Here's how the part is built. I have some questions about the finished solid (model axes, mm). A direction names the side the tool comes from. Give positions to 0.01 mm unless a question says otherwise; leave off trailing zeros. Write each loop counter-clockwise with the first axis right and the second up, starting at its lowest first coordinate (ties: lowest second). Pieces come first, ordered by that corner, then holes. Notation, with made-up numbers: (-5.5, 42) - (50.5, 42) arc R19 cw to (50.5, 60) - close; hole circle Ø9 at (36, 22). An arc over 180 degrees is marked (long way). Use a Markdown table: item, result.
```python
from build123d import *

# Parameters (mm, degrees)
F1_DEPTH  = 270
F2_W      = 88
F2_H      = 212
F3_DEPTH  = 178
F4_W      = 68
F4_H      = 172
F5_DEPTH  = 5
F7_DEPTH  = 128
F8_W      = 42
F8_H      = 66
F9_DEPTH  = 163
F11_DEPTH = 146


with BuildPart() as f1:
    # F0 (on Front) → F1 (new body)
    with BuildSketch(Plane.XZ):
        with BuildLine():
            Line((-20, 505), (-665, 505))
            ThreePointArc((-665, 505), (-679.142136, 499.142136), (-685, 485))
            Line((-685, 485), (-685, 20))
            ThreePointArc((-685, 20), (-679.142136, 5.857864), (-665, 0))
            Line((-665, 0), (-20, 0))
            ThreePointArc((-20, 0), (-5.857864, 5.857864), (0, 20))
            Line((0, 20), (0, 485))
            ThreePointArc((0, 485), (-5.857864, 499.142136), (-20, 505))
        make_face()
    extrude(amount=-F1_DEPTH)

    # F2 (on face) → F3 (cut)
    with BuildSketch(Plane.XZ):
        with Locations((-541.250854, 142.595568)):
            Rectangle(F2_W, F2_H)
    extrude(amount=-F3_DEPTH, mode=Mode.SUBTRACT)

    # F4 (on face) → F5 (cut)
    with BuildSketch(Plane.XZ.offset(-178)):
        with Locations((-541.250854, 142.595568)):
            Rectangle(F4_W, F4_H)
    extrude(amount=-F5_DEPTH, mode=Mode.SUBTRACT)

    # F6 (on face) → F7 (cut)
    with BuildSketch(Plane.XZ):
        with BuildLine():
            Line((-456.298642, 342.595568), (-456.298642, 36.595568))
            Line((-456.298642, 36.595568), (-279.298642, 36.595568))
            Line((-279.298642, 36.595568), (-271.298642, 36.595568))
            ThreePointArc((-271.298642, 36.595568), (-269.884428, 37.181354), (-269.298642, 38.595568))
            Line((-269.298642, 38.595568), (-269.298642, 61.595568))
            ThreePointArc((-269.298642, 61.595568), (-269.884428, 63.009782), (-271.298642, 63.595568))
            Line((-271.298642, 63.595568), (-277.298642, 63.595568))
            ThreePointArc((-277.298642, 63.595568), (-278.712855, 64.181354), (-279.298642, 65.595568))
            Line((-279.298642, 65.595568), (-279.298642, 313.595568))
            ThreePointArc((-279.298642, 313.595568), (-278.712855, 315.009782), (-277.298642, 315.595568))
            Line((-277.298642, 315.595568), (-271.298642, 315.595568))
            ThreePointArc((-271.298642, 315.595568), (-269.884428, 316.181354), (-269.298642, 317.595568))
            Line((-269.298642, 317.595568), (-269.298642, 340.595568))
            ThreePointArc((-269.298642, 340.595568), (-269.884428, 342.009782), (-271.298642, 342.595568))
            Line((-271.298642, 342.595568), (-317.298642, 342.595568))
            Line((-317.298642, 342.595568), (-317.298642, 402.595568))
            ThreePointArc((-317.298642, 402.595568), (-320.227574, 409.666636), (-327.298642, 412.595568))
            Line((-327.298642, 412.595568), (-396.298642, 412.595568))
            ThreePointArc((-396.298642, 412.595568), (-403.36971, 409.666636), (-406.298642, 402.595568))
            Line((-406.298642, 402.595568), (-406.298642, 342.595568))
            Line((-406.298642, 342.595568), (-456.298642, 342.595568))
        make_face()
    extrude(amount=-F7_DEPTH, mode=Mode.SUBTRACT)

    # F8 (on face) → F9 (cut)
    with BuildSketch(Plane.XZ):
        with Locations((-171, 68.898773)):
            Rectangle(F8_W, F8_H)
    extrude(amount=-F9_DEPTH, mode=Mode.SUBTRACT)

    # F10 (on face) → F11 (cut)
    with BuildSketch(Plane.XZ):
        Polygon((-192, 275.058829), (-192, 176.058829), (-138, 176.058829), (-138, 206.058829), (-158, 206.058829), (-158, 275.058829), align=None)
    extrude(amount=-F11_DEPTH, mode=Mode.SUBTRACT)


solid = f1.part
```
Item 1: For faces 4 (the cylindrical face through (-678.986, 133.11, 499.297)), 5 (the flat face through (-406.299, 63, 373)), which set-ups out of +Z, -Z, +X, -X, +Y, -Y let a thin tool reach every point of the face, with its end or its side?
Values:
| item | result |
|---|---|
| face 4 | +Z, -X, +Y, -Y |
| face 5 | -Y |
Item 2: If we section it at A-A, the plane z = 299.5: Write out the boundary of the cut face in (x, y), plus the area to 3 significant figures.
Values:
| item | result |
|---|---|
| outline | (-685, 0) - (-456.3, 0) - (-456.3, 128) - (-279.3, 128) - (-279.3, 0) - (0, 0) - (0, 270) - (-685, 270) - close |
| area | 162,000 mm2 |
Item 3: I need wall thicknesses on line 1 along X through (y, z) = (16.5, 130); line 2 along X through (y, z) = (104.5, 87); line 3 along Z through (x, y) = (-186, 65.5). Which ranges of each line are inside material? Lowest first, please. Write a range as [from, to].
Values:
| item | result |
|---|---|
| line 1 | x = [-685, -585.25], [-497.25, -456.3], [-279.3, 0] |
| line 2 | x = [-685, -585.25], [-497.25, -456.3], [-279.3, -192], [-150, 0] |
| line 3 | z = [0, 35.9], [101.9, 176.06], [275.06, 505] |
Item 4: If we section it at B-B, the plane y = 100: Count the separate pieces of the cut face and the enclosed holes in it, plus the area to 3 significant figures.
Values:
| item | result |
|---|---|
| separate pieces | 1 |
| enclosed holes | 4 |
| area | 259,000 mm2 |
Item 5: Will this pin go through, and if not, where does the flat tip stop? pin 1 Ø5 at (x, z) = (-301.5, 284.5) entering from -Y.
Values:
| item | result |
|---|---|
| pin 1 | stops at y = 128 |
Item 6: If we section it at D-D, the plane z = 360.5: Write out the boundary of the cut face in (x, y).
Values:
| item | result |
|---|---|
| outline | (-685, 0) - (-406.3, 0) - (-406.3, 128) - (-317.3, 128) - (-317.3, 0) - (0, 0) - (0, 270) - (-685, 270) - close |
Item 7: If we section it at C-C, the plane z = 78.5: Write out the boundary of the cut face in (x, y).
Values:
| item | result |
|---|---|
| outline | (-685, 0) - (-585.25, 0) - (-585.25, 178) - (-575.25, 178) - (-575.25, 183) - (-507.25, 183) - (-507.25, 178) - (-497.25, 178) - (-497.25, 0) - (-456.3, 0) - (-456.3, 128) - (-279.3, 128) - (-279.3, 0) - (-192, 0) - (-192, 163) - (-150, 163) - (-150, 0) - (0, 0) - (0, 270) - (-685, 270) - close |
Item 8: Thinking about a two-plate mould opening in Z: for faces 1 (the flat face through (-685, 133, 256)), 2 (the flat face through (-171, 146, 226)), 3 (the cylindrical face through (-5.703, 133.11, 498.986)), which applies, +Z half, -Z half, draft (parallel to the pull), parting line (faces both ways), or undercut?
Values:
| item | result |
|---|---|
| face 1 | draft |
| face 2 | undercut |
| face 3 | +Z half |
